Source: CAD feature listing. Evaluate the final solid. Frame: model axes, mm. A direction names the side the tool comes from. Coordinates: 2 decimals unless noted, no trailing zeros. Loops run counter-clockwise (first coordinate to the right, second up) from the corner with the lowest first, then second, coordinate; pieces in that order, holes last. Notation, with made-up numbers: (14.25, 84) -> (65.25, 84) arc R36 ccw to (65.25, 120) -> close; hole circle Ø3 at (62, 49). An arc over 180 degrees is marked (long way). Answer as a JSON object with one key per item and string values. Group by question number.
from build123d import *

# Parameters (mm, degrees)
SOCKET_1_SKETCH_W = 15
SOCKET_1_SKETCH_H = 5.5


with BuildPart() as part:
    # CV_Nuvair Sketch → CV_Nuvair (revolve)
    with BuildSketch(Plane.XY, mode=Mode.PRIVATE) as cv_nuvair_sk:
        Polygon((12.7, 0), (12.7, 5.5), (0, 5.5), (0, 12.7), (-48.3, 12.7), (-48.3, 0), align=None)
    revolve(cv_nuvair_sk.sketch.rotate(Axis((-1000, 0, 0), (1, 0, 0)), 90), axis=Axis((-1000, 0, 0), (1, 0, 0)))

    # Socket 1 Sketch → Socket 1 (revolve, cut)
    with BuildSketch(Plane.XY, mode=Mode.PRIVATE) as socket_1_sk:
        with Locations((-41.8, 2.75)):
            Rectangle(SOCKET_1_SKETCH_W, SOCKET_1_SKETCH_H)
    revolve(socket_1_sk.sketch.rotate(Axis((-1000, 0, 0), (1, 0, 0)), 90), axis=Axis((-1000, 0, 0), (1, 0, 0)), mode=Mode.SUBTRACT)


solid = part.part
1. Section query B-B on y = 0. Return loops of the section in (x, z), then the cut area to 3 significant figures.
2. Section query A-A on x = -43. Return loops of the section in (y, z), then the cut area to 3 significant figures.
3. Reachability of faces 5 (the face through (12.7, 0, 0)), 6 (the face through (0, 3, -5)) from +Z, -Z, +X, -X, +Y, -Y: full face, straight path, thin tool, end or side. Return the list, or none.
4. Ray query, L1, parallel to X at y = 5.5, z = -3.75; L2, parallel to X at y = -3.5, z = -1.5; L3, parallel to Y at x = -39, z = 5. Return the intervals inside material, ascending.
5. Mould query, pull axis Z, two halves, no side actions, for faces 1 (the face through (-48.3, 3, 5)), 2 (the face through (-34.3, 0, 0)), 3 (the face through (-41.2, 5.37, -1.19)), 4 (the face through (6.26, 5.37, -1.19)). Classes: pulls with the +Z half, pulls with the -Z half, needs draft (parallel to the pull), parting line crosses it, or undercut.
6. Section query D-D on x = -3. Return loops of the section in (y, z), then the cut area to 3 significant figures.
7. Pin query (flat end, axial travel): pin 1 Ø5.5 at (y, z) = (-1.5, 1) entering from -X; pin 2 Ø1.5 at (x, z) = (-18.5, -9) entering from -Y; pin 3 Ø5 at (x, y) = (-20.5, -9) entering from +Z. Return the tip coordinate at first contact, or that it passes through.
Solved:
{
 "1": {"outline": "(-48.3, -12.7) -> (0, -12.7) -> (0, -5.5) -> (12.7, -5.5) -> (12.7, 5.5) -> (0, 5.5) -> (0, 12.7) -> (-48.3, 12.7) -> (-48.3, 5.5) -> (-34.3, 5.5) -> (-34.3, -5.5) -> (-48.3, -5.5) -> close", "area": "1,210 mm^2"},
 "2": {"outline": "circle Ø25.4 at (0, 0); hole circle Ø11 at (0, 0)", "area": "412 mm^2"},
 "3": {"face 5": "+Z, -Z, +X, +Y, -Y", "face 6": "+X"},
 "4": {"L1": "-48.3 to 0", "L2": "-34.3 to 12.7", "L3": "-11.67 to -2.29, 2.29 to 11.67"},
 "5": {"face 1": "needs draft", "face 2": "undercut", "face 3": "undercut", "face 4": "parting line crosses it"},
 "6": {"outline": "circle Ø25.4 at (0, 0)", "area": "507 mm^2"},
 "7": {"pin 1": "x = -34.3", "pin 2": "y = -9.66", "pin 3": "z = 10.91"}
}
